Source: CAD feature listing. Evaluate the final solid. Frame: model axes, mm. Round coordinates to 2 decimals unless told otherwise and drop trailing zeros. Order: outer loops, then holes, each group sorted by start corner. A loop starts at its lowest first (then second) coordinate and runs counter-clockwise, first axis right, second up. Notation, with made-up numbers: M -33,-28 L 24,-28 A15 cw 24,-20 Z; hole C 71.5,83 d11. An arc over 180 degrees is marked long. Answer as CSV lines item,"result". Start each with the question number.
Item 1: Section query C-C on y = -8. Return the cut outline in (x, z).
Item 2: Section query A-A on y = 0. Return the cut outline in (x, z), plus the area to 3 significant figures.
Item 3: Line query: line 1 (Y direction, x = 6, z = 0.5); line 2 (X direction, y = 3, z = -18); line 3 (X direction, y = 1, z = -22.5). Output: solid intervals per line, ascending. Write a range as [from, to].
Item 4: Pull-direction query (Z, two-part tool) for faces 1 (the face through (0, -15, 0)), 2 (the face through (-23, 0, 0)), 3 (the face through (0, 0, 30)); classes: +Z half, -Z half, draft (parallel to the pull), parting line (faces both ways), or undercut.
Item 5: Section query B-B on z = -20.5. Return the cut outline in (x, y), plus the area to 3 significant figures.
Item 6: Section query D-D on y = 3.75. Return the cut outline in (x, z).
Item 7: First-contact query: P1, Ø3, axis at y = -9.5, z = -19, coming from the -X side; P2, Ø10.5, axis at x = 6.19, y = 0, coming from the -Z side; P3, Ø4, axis at y = 5, z = -2, coming from the +X side; P4, Ø5, axis at y = -1, z = -23, coming from the +X side. Flat tips, straight axial feed; report the tip coordinate or a pass-through.
from build123d import *

# Parameters (mm, degrees)
F1_DEPTH      = 15
F1_DEPTH_BACK = 15
F2_R          = 4.554576
F3_DEPTH      = 65.6


with BuildPart() as f1:
    # F0 (on Front) → F1 (new body, two sides)
    with BuildSketch(Plane.XZ) as f1_sk:
        Polygon((30, 30), (-14.883985, 30), (-1.883985, -30), (16, -30), align=None)
        Polygon((-14.883985, 30), (-25.116015, 30), (-12.116015, -30), (-1.883985, -30), align=None)
        Polygon((-25.116015, 30), (-30, 30), (-16, -30), (-12.116015, -30), align=None)
    extrude(amount=F1_DEPTH)
    extrude(f1_sk.sketch, amount=-F1_DEPTH_BACK)

    # F2 (on face) → F3 (cut)
    with BuildSketch(Plane(origin=(0, 0, -30), x_dir=(1, 0, 0), z_dir=(0, 0, -1))):
        with Locations((6.190634, 0)):
            Circle(F2_R)
    extrude(amount=-F3_DEPTH, mode=Mode.SUBTRACT)


solid = f1.part
Results:
1,outline,"M -30,30 L -16,-30 L 16,-30 L 30,30 Z"
2,outline,"M -30,30 L -16,-30 L 1.64,-30 L 1.64,30 Z; M 10.75,-30 L 16,-30 L 30,30 L 10.75,30 Z"
2,area,"2,210 mm^2"
3,line 1,"[-15, -4.55], [4.55, 15]"
3,line 2,"[-18.8, 2.76], [9.62, 18.8]"
3,line 3,"[-17.75, 1.75], [10.63, 17.75]"
4,face 1,"draft"
4,face 2,"-Z half"
4,face 3,"+Z half"
5,outline,"M -18.22,-15 L 18.22,-15 L 18.22,15 L -18.22,15 Z; hole C 6.19,0 d9.11"
5,area,"1,030 mm^2"
6,outline,"M -30,30 L -16,-30 L 3.61,-30 L 3.61,30 Z; M 8.78,-30 L 16,-30 L 30,30 L 8.78,30 Z"
7,P1,"x = -18.92"
7,P2,"z = -30"
7,P3,"x = 23"
7,P4,"x = 18.22"
